```python
from build123d import *

# Parameters (mm, degrees)
F0_R     = 152.4
F0_R_2   = 38.1
F1_DEPTH = 38.1
F2_R     = 12.7
F3_DEPTH = 19.05
F4_R     = 12.7
F5_DEPTH = 6.35


with BuildPart() as f1:
    # F0 (on Front) → F1 (new body)
    with BuildSketch(Plane.XZ):
        with Locations((-14.28063, 39.245158)):
            Circle(F0_R)
        with BuildLine():
            ThreePointArc((65.410439, 138.130615), (100.283251, 94.054985), (112.71937, 39.245158))
            ThreePointArc((112.71937, 39.245158), (111.613264, 22.520101), (108.314212, 6.086378))
            ThreePointArc((108.314212, 6.086378), (111.593745, 3.796365), (112.853548, 0))
            ThreePointArc((112.853548, 0), (110.171472, -5.183516), (104.390923, -5.988265))
            ThreePointArc((104.390923, -5.988265), (60.368097, -63.5), (-7.932614, -87.596092))
            ThreePointArc((-7.932614, -87.596092), (-7.931126, -87.675461), (-7.93063, -87.754842))
            ThreePointArc((-7.93063, -87.754842), (-14.360011, -94.104346), (-20.628645, -87.596092))
            ThreePointArc((-20.628645, -87.596092), (-88.929357, -63.5), (-132.952182, -5.988265))
            ThreePointArc((-132.952182, -5.988265), (-141.104016, -1.962258), (-136.875472, 6.086378))
            ThreePointArc((-136.875472, 6.086378), (-135.064807, 78.490317), (-93.971698, 138.130615))
            ThreePointArc((-93.971698, 138.130615), (-92.661793, 147.127574), (-83.700394, 145.593155))
            ThreePointArc((-83.700394, 145.593155), (-14.28063, 166.245158), (55.139134, 145.593155))
            ThreePointArc((55.139134, 145.593155), (62.254706, 148.053584), (66.718097, 141.990317))
            ThreePointArc((66.718097, 141.990317), (66.382304, 139.952716), (65.410439, 138.130615))
        make_face(mode=Mode.SUBTRACT)
        with BuildLine():
            ThreePointArc((108.314212, 6.086378), (111.613264, 22.520101), (112.71937, 39.245158))
            ThreePointArc((112.71937, 39.245158), (100.283251, 94.054985), (65.410439, 138.130615))
            ThreePointArc((65.410439, 138.130615), (56.635661, 136.853059), (55.139134, 145.593155))
            ThreePointArc((55.139134, 145.593155), (-14.28063, 166.245158), (-83.700394, 145.593155))
            ThreePointArc((-83.700394, 145.593155), (-82.86609, 143.876925), (-82.579357, 141.990317))
            ThreePointArc((-82.579357, 141.990317), (-86.891756, 135.97611), (-93.971698, 138.130615))
            ThreePointArc((-93.971698, 138.130615), (-135.064807, 78.490317), (-136.875472, 6.086378))
            ThreePointArc((-136.875472, 6.086378), (-131.268442, 5.090197), (-128.714807, 0))
            ThreePointArc((-128.714807, 0), (-129.881292, -3.667924), (-132.952182, -5.988265))
            ThreePointArc((-132.952182, -5.988265), (-88.929357, -63.5), (-20.628645, -87.596092))
            ThreePointArc((-20.628645, -87.596092), (-14.28063, -81.404842), (-7.932614, -87.596092))
            ThreePointArc((-7.932614, -87.596092), (60.368097, -63.5), (104.390923, -5.988265))
            ThreePointArc((104.390923, -5.988265), (100.464339, 1.962258), (108.314212, 6.086378))
        make_face()
        with BuildLine():
            ThreePointArc((84.119287, 64.543705), (86.516175, 51.995227), (87.31937, 39.245158))
            ThreePointArc((87.31937, 39.245158), (77.64284, -4.028803), (50.456462, -39.059816))
            ThreePointArc((50.456462, -39.059816), (51.446159, -40.894576), (51.788352, -42.950968))
            ThreePointArc((51.788352, -42.950968), (47.305996, -49.020104), (40.186964, -46.521042))
            ThreePointArc((40.186964, -46.521042), (-14.28063, -62.354842), (-68.748224, -46.521042))
            ThreePointArc((-68.748224, -46.521042), (-77.732048, -48.088226), (-79.017722, -39.059816))
            ThreePointArc((-79.017722, -39.059816), (-110.907972, 7.849032), (-112.680546, 64.543705))
            ThreePointArc((-112.680546, 64.543705), (-116.947181, 72.603543), (-108.757947, 76.616224))
            ThreePointArc((-108.757947, 76.616224), (-73.999611, 121.441285), (-20.627528, 140.646721))
            ThreePointArc((-20.627528, 140.646721), (-14.379861, 147.194383), (-7.93063, 140.845158))
            ThreePointArc((-7.93063, 140.845158), (-7.931405, 140.745927), (-7.933731, 140.646721))
            ThreePointArc((-7.933731, 140.646721), (45.438352, 121.441285), (80.196688, 76.616224))
            ThreePointArc((80.196688, 76.616224), (85.998414, 75.836242), (88.696712, 70.641285))
            ThreePointArc((88.696712, 70.641285), (87.425017, 66.829025), (84.119287, 64.543705))
        make_face(mode=Mode.SUBTRACT)
        with BuildLine():
            ThreePointArc((50.456462, -39.059816), (77.64284, -4.028803), (87.31937, 39.245158))
            ThreePointArc((87.31937, 39.245158), (86.516175, 51.995227), (84.119287, 64.543705))
            ThreePointArc((84.119287, 64.543705), (76.307504, 68.679027), (80.196688, 76.616224))
            ThreePointArc((80.196688, 76.616224), (45.438352, 121.441285), (-7.933731, 140.646721))
            ThreePointArc((-7.933731, 140.646721), (-14.28063, 134.495158), (-20.627528, 140.646721))
            ThreePointArc((-20.627528, 140.646721), (-73.999611, 121.441285), (-108.757947, 76.616224))
            ThreePointArc((-108.757947, 76.616224), (-105.713015, 74.292986), (-104.557972, 70.641285))
            ThreePointArc((-104.557972, 70.641285), (-107.095712, 65.562981), (-112.680546, 64.543705))
            ThreePointArc((-112.680546, 64.543705), (-110.907972, 7.849032), (-79.017722, -39.059816))
            ThreePointArc((-79.017722, -39.059816), (-71.943219, -36.943161), (-67.649611, -42.950968))
            ThreePointArc((-67.649611, -42.950968), (-67.930476, -44.818612), (-68.748224, -46.521042))
            ThreePointArc((-68.748224, -46.521042), (-14.28063, -62.354842), (40.186964, -46.521042))
            ThreePointArc((40.186964, -46.521042), (41.705916, -37.81371), (50.456462, -39.059816))
        make_face()
        with Locations((-14.28063, 39.245158)):
            Circle(F0_R_2, mode=Mode.SUBTRACT)
    extrude(amount=F1_DEPTH)

    # F2 (on face) → F3 (cut)
    with BuildSketch(Plane(origin=(0, 0, 0), x_dir=(-1, 0, 0), z_dir=(0, 1, 0))):
        with Locations((14.28063, 140.845158)):
            Circle(F2_R)
        with Locations((-82.346712, 70.641285)):
            Circle(F2_R)
        with Locations((-45.438352, -42.950968)):
            Circle(F2_R)
        with Locations((73.999611, -42.950968)):
            Circle(F2_R)
        with Locations((110.907972, 70.641285)):
            Circle(F2_R)
    extrude(amount=-F3_DEPTH, mode=Mode.SUBTRACT)

    # F4 (on face) → F5 (cut)
    with BuildSketch(Plane.XZ.offset(38.1)):
        with Locations((-88.929357, 141.990317)):
            Circle(F4_R)
        with Locations((-135.064807, 0)):
            Circle(F4_R)
        with Locations((-14.28063, -87.754842)):
            Circle(F4_R)
        with Locations((106.503548, 0)):
            Circle(F4_R)
        with Locations((60.368097, 141.990317)):
            Circle(F4_R)
    extrude(amount=-F5_DEPTH, mode=Mode.SUBTRACT)


solid = f1.part
```
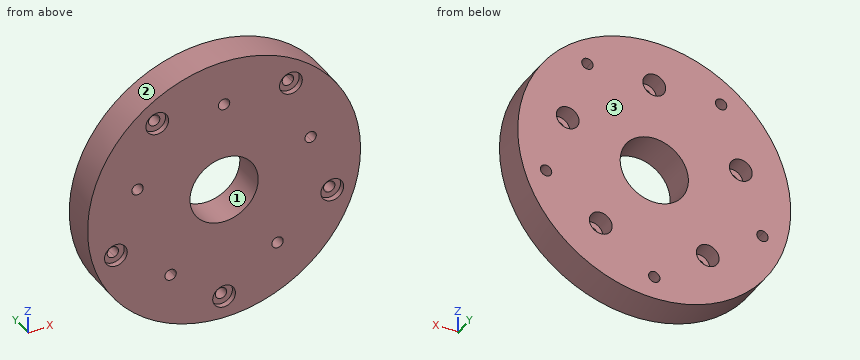
Input: part model. Units: mm. Frame: model coordinates. Face numbers are marked on the shaded views. Round coordinates to 2 decimals unless told otherwise and drop trailing zeros. Order: outer loops, then holes, each group sorted by start corner. A loop starts at its lowest first (then second) coordinate and runs counter-clockwise, first axis right, second up. Notation, with made-up numbers: (69.25, 89.25) - (126.25, 89.25) arc R18 ccw to (126.25, 103.25) - close; hole circle Ø9 at (-38.75, 9). An arc over 180 degrees is marked (long way). Answer in a Markdown table with one row per item.
Item 1: Pin query (flat end, axial travel): pin 1 (2 mm diameter, centred on x = -35.5, y = -23.5, fed in from -Z); pin 2 (1.5 mm diameter, centred on x = -5.5, y = -18, fed in from -Z); pin 3 (7.5 mm diameter, centred on x = 104.5, z = 0.5, fed in from -Y); pin 4 (10 mm diameter, centred on x = 61.5, y = -5, fed in from +Z). Return the tip coordinate at first contact, or that it passes through.
Model answer:
| item | result |
|---|---|
| pin 1 | stops at z = -111.81 |
| pin 2 | stops at z = -112.94 |
| pin 3 | passes through |
| pin 4 | stops at z = 174.21 |
Item 2: Section query B-B (y = -15). Give the number of separate pieces and of enclosed holes in the cut face, then the cut area to 3 significant figures.
Model answer:
| item | result |
|---|---|
| separate pieces | 1 |
| enclosed holes | 11 |
| area | 65,200 mm² |
Item 3: Mould query, pull axis Z, two halves, no side actions, for the marked faces 1, 2 and 3. Classes: released by +Z, released by -Z, zero draft, split by the parting line, or undercut.
Model answer:
| item | result |
|---|---|
| face 1 | undercut |
| face 2 | split by the parting line |
| face 3 | zero draft |
Item 4: Line query: line 1 (Z direction, x = -85, y = -8.5); line 2 (Z direction, x = 73.5, y = -13); line 3 (X direction, y = -24, z = 29). Output: solid intervals per line, ascending.
Model answer:
| item | result |
|---|---|
| line 1 | z = -95.75 to -49.3, -36.6 to 137, 146.98 to 174.24 |
| line 2 | z = -85.34 to 61.53, 79.75 to 163.83 |
| line 3 | x = -166.34 to -50.98, 22.42 to 137.77 |
Item 5: Section query C-C (z = -18). Return the cut outline in (x, y), then the cut area to 3 significant figures.
Model answer:
| item | result |
|---|---|
| outline | (-155.52, -38.1) - (126.96, -38.1) - (126.96, 0) - (-155.52, 0) - close |
| area | 10,800 mm² |
Item 6: Section query A-A (z = 22). Return the cut outline in (x, y).
Model answer:
| item | result |
|---|---|
| outline | (-165.7, -38.1) - (-48.25, -38.1) - (-48.25, 0) - (-165.7, 0) - close; (19.69, -38.1) - (137.14, -38.1) - (137.14, 0) - (19.69, 0) - close |
